Could you check a few things on this model? Use its own coordinates, in mm. Face numbers are marked on the shaded views. Give positions to 0.01 mm unless a question says otherwise; leave off trailing zeros. Write each loop counter-clockwise with the first axis right and the second up, starting at its lowest first coordinate (ties: lowest second). Pieces come first, ordered by that corner, then holes. Notation, with made-up numbers: (20.25, 50.5) - (65.25, 50.5) arc R21 ccw to (65.25, 65.5) - close; hole circle Ø11 at (3.5, 79). An arc over 180 degrees is marked (long way). Write item = value, one per line.
from build123d import *

# Parameters (mm, degrees)
BASE_FLANGE1_DEPTH = 1
EDGE_FLANGE1_DEPTH = 24
HEM1_START         = -12
HEM1_DEPTH         = 24
HEM1_2_DEPTH       = 24
CUT_EXTRUDE1_DEPTH = 10


# Read off the part's stored shape, not the designer's step: Hem1
# Sheet-metal steps are written as plain solids
with BuildPart() as part:
    # Sketch1 → Base-Flange1 (new body)
    with BuildSketch(Plane(origin=(0, 0, 0), x_dir=(1, 0, 0), z_dir=(0, 1, 0))):
        with BuildLine():
            Line((0, 12), (9, 12))
            Line((9, 12), (23.322209849, 7.655543182))
            ThreePointArc((23.322209849, 7.655543182), (29, 0), (23.322209849, -7.655543182))
            Line((23.322209849, -7.655543182), (9, -12))
            Line((9, -12), (0, -12))
            Line((0, -12), (0, 12))
        make_face()
        with BuildLine():
            Line((14, 2), (16.527864045, 2))
            ThreePointArc((16.527864045, 2), (17.344360626, 2.174258142), (18.01857603, 2.666666667))
            ThreePointArc((18.01857603, 2.666666667), (25, 0), (18.01857603, -2.666666667))
            ThreePointArc((18.01857603, -2.666666667), (17.344360626, -2.174258142), (16.527864045, -2))
            Line((16.527864045, -2), (14, -2))
            ThreePointArc((14, -2), (12, 0), (14, 2))
        make_face(mode=Mode.SUBTRACT)
    extrude(amount=-BASE_FLANGE1_DEPTH)

    # Edge-Flange1 section (across the edge) → Edge-Flange1 (add)
    with BuildSketch(Plane(origin=(-1, 0, -12), x_dir=(1, 0, 0), z_dir=(0, 0, 1))):
        with BuildLine():
            Line((-1, 1), (-1, 20))
            Line((-1, 20), (0, 20))
            Line((0, 20), (0, 1))
            ThreePointArc((0, 1), (0.292893219, 0.292893219), (1, 0))
            Line((1, 0), (1, -1))
            ThreePointArc((1, -1), (-0.414213562, -0.414213562), (-1, 1))
        make_face()
    extrude(amount=EDGE_FLANGE1_DEPTH)

    # Hem1 outline → Hem1 (cut)
    with BuildSketch(Plane.XY.offset(HEM1_START)):
        with BuildLine():
            ThreePointArc((-2, 18.95), (-1.709934208, 19.674568837), (-1, 19.998808848))
            Line((-1, 19.998808848), (-1, 20))
            Line((-1, 20), (-2, 20))
            Line((-2, 20), (-2, 18.95))
        make_face()
    extrude(amount=HEM1_DEPTH, mode=Mode.SUBTRACT)

    # Hem1 2 outline → Hem1 2 (add)
    with BuildSketch(Plane.XY.offset(HEM1_START)):
        with BuildLine():
            Line((-0.9, 16), (0.1, 16))
            Line((0.1, 16), (0.1, 18.95))
            ThreePointArc((0.1, 18.95), (-0.225431163, 19.709934208), (-1, 19.998808848))
            Line((-1, 19.998808848), (-1, 18.95))
            ThreePointArc((-1, 18.95), (-0.95, 19), (-0.9, 18.95))
            Line((-0.9, 18.95), (-0.9, 16))
        make_face()
    extrude(amount=HEM1_2_DEPTH)

    # Sketch13 → Cut-Extrude1 (cut)
    with BuildSketch(Plane(origin=(-1, 0, 0), x_dir=(0, 0, -1), z_dir=(1, 0, 0))):
        with BuildLine():
            Line((-5, 14), (5, 14))
            ThreePointArc((5, 14), (5.707106781, 13.707106781), (6, 13))
            Line((6, 13), (6, 5))
            ThreePointArc((6, 5), (5.707106781, 4.292893219), (5, 4))
            Line((5, 4), (-5, 4))
            ThreePointArc((-5, 4), (-5.707106781, 4.292893219), (-6, 5))
            Line((-6, 5), (-6, 13))
            ThreePointArc((-6, 13), (-5.707106781, 13.707106781), (-5, 14))
        make_face()
    extrude(amount=-CUT_EXTRUDE1_DEPTH, mode=Mode.SUBTRACT)


solid = part.part
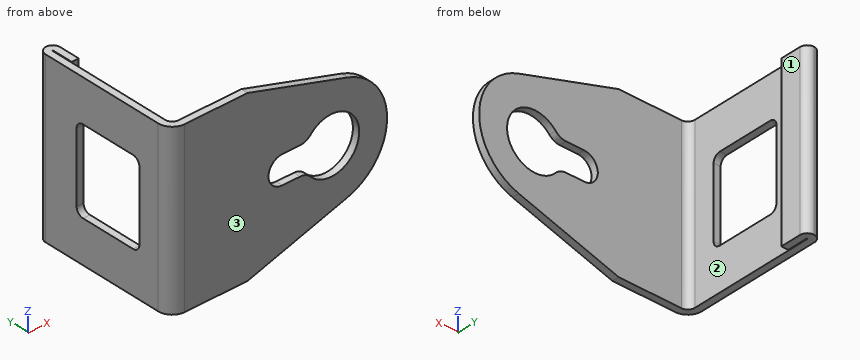
1. For pin 1 (12 mm diameter, centred on x = 15, z = -5, fed in from +Y); pin 2 (1.1 mm diameter, centred on x = 15.5, y = -0.5, fed in from -Z); pin 3 (1 mm diameter, centred on y = 8, z = -5, fed in from +X); pin 4 (0.5 mm diameter, centred on x = 16, y = -0.5, fed in from +Z), each with a flat end and sliding along its axis, tell me the tip position at first contact or that it passes through.
Filled sheet:
pin_1 = 0
pin_2 = -10.2
pin_3 = through
pin_4 = 9.95
2. If we section it at A-A, the plane y = 17.75: Please give me the cut outline in (x, z), and give its area (3 significant figures).
Filled sheet:
outline = (-2, -12) - (-1, -12) - (-1, 12) - (-2, 12) - close; (-0.9, -12) - (0.1, -12) - (0.1, 12) - (-0.9, 12) - close
area = 48.0 mm2
3. I need wall thicknesses on line 1 (Y direction, x = 12.5, z = -8.5); line 2 (X direction, y = 2.25, z = 10.5); line 3 (Z direction, x = 21, y = -0.45). Which ranges of each line are inside material? Lowest first, please.
Filled sheet:
line_1 = -1 to 0
line_2 = -2 to -1
line_3 = -8.36 to -4, 4 to 8.36
4. If we section it at C-C, the plane x = 21: Please give me the cut outline in (y, z), and give its area (3 significant figures).
Filled sheet:
outline = (-1, -8.36) - (0, -8.36) - (0, -4) - (-1, -4) - close; (-1, 4) - (0, 4) - (0, 8.36) - (-1, 8.36) - close
area = 8.72 mm2
5. Thinking about a two-plate mould opening in Y: for the marked faces 1, 2 and 3, which applies, pulls with the +Y half, pulls with the -Y half, needs draft (parallel to the pull), parting line crosses it, or undercut?
Filled sheet:
face_1 = needs draft
face_2 = undercut
face_3 = pulls with the -Y half
6. If we section it at B-B, the plane z = 0: Please give me the cut outline in (x, y).
Filled sheet:
outline = (-2, 1) arc R2 ccw to (0, -1) - (12, -1) - (12, 0) - (0, 0) arc R1 cw to (-1, 1) - (-1, 4) - (-2, 4) - close; (-2, 14) - (-1, 14) - (-1, 18.95) arc R0.05 cw to (-0.9, 18.95) - (-0.9, 16) - (0.1, 16) - (0.1, 18.95) arc R1.05 ccw to (-2, 18.95) - close; (25, -1) - (29, -1) - (29, 0) - (25, 0) - close
7. If we section it at D-D, the plane z = -3.5: Please give me the cut outline in (x, y).
Filled sheet:
outline = (-2, 1) arc R2 ccw to (0, -1) - (19.06, -1) - (19.06, 0) - (0, 0) arc R1 cw to (-1, 1) - (-1, 4) - (-2, 4) - close; (-2, 14) - (-1, 14) - (-1, 18.95) arc R0.05 cw to (-0.9, 18.95) - (-0.9, 16) - (0.1, 16) - (0.1, 18.95) arc R1.05 ccw to (-2, 18.95) - close; (22.94, -1) - (28.19, -1) - (28.19, 0) - (22.94, 0) - close
